The listing builds one solid part. Answer for the finished solid, in the listing's coordinates (mm). A direction names the side the tool comes from. Coordinates: 2 decimals unless noted, no trailing zeros. Order: outer loops, then holes, each group sorted by start corner. A loop starts at its lowest first (then second) coordinate and runs counter-clockwise, first axis right, second up. Notation, with made-up numbers: (-6, 23) -> (22, 23) arc R27 cw to (22, 50) -> close; hole circle Ø8 at (-23.75, 64.25). An arc over 180 degrees is marked (long way). Answer in a Markdown table with one row per item. Add a question column.
```python
from build123d import *

# Parameters (mm, degrees)
SKETCH1_W           = 88
SKETCH1_H           = 82
BOSS_EXTRUDE1_DEPTH = 3
SKETCH2_R           = 1.7
CUT_EXTRUDE1_DEPTH  = 4
SKETCH4_W           = 81.2
SKETCH4_H           = 75.2
SKETCH4_W_2         = 75.2
SKETCH4_H_2         = 69.2
BOSS_EXTRUDE2_DEPTH = 2
CUT_EXTRUDE5_START  = -3
SKETCH6_R           = 6
CUT_EXTRUDE5_DEPTH  = 3
SKETCH7_W           = 88
SKETCH7_H           = 3
BOSS_EXTRUDE3_DEPTH = 4
SKETCH8_R           = 3.75
BOSS_EXTRUDE4_DEPTH = 3


with BuildPart() as part:
    # Sketch1 → Boss-Extrude1 (new body)
    with BuildSketch(Plane(origin=(0, 0, 0), x_dir=(1, 0, 0), z_dir=(0, 1, 0))):
        Rectangle(SKETCH1_W, SKETCH1_H)
    extrude(amount=BOSS_EXTRUDE1_DEPTH)

    # Sketch2 → Cut-Extrude1 (cut, through all)
    with BuildSketch(Plane(origin=(0, 3, 0), x_dir=(1, 0, 0), z_dir=(0, 1, 0))):
        with Locations((-38, 35)):
            Circle(SKETCH2_R)
        with Locations((38, 35)):
            Circle(SKETCH2_R)
        with Locations((38, -35)):
            Circle(SKETCH2_R)
        with Locations((-38, -35)):
            Circle(SKETCH2_R)
    extrude(amount=-CUT_EXTRUDE1_DEPTH, mode=Mode.SUBTRACT)

    # Sketch4 → Boss-Extrude2 (add)
    with BuildSketch(Plane.XZ):
        Rectangle(SKETCH4_W, SKETCH4_H)
        Rectangle(SKETCH4_W_2, SKETCH4_H_2, mode=Mode.SUBTRACT)
    extrude(amount=BOSS_EXTRUDE2_DEPTH)

    # Sketch6 → Cut-Extrude5 (cut, through all)
    with BuildSketch(Plane(origin=(0, 3, 0), x_dir=(1, 0, 0), z_dir=(0, 1, 0)).offset(CUT_EXTRUDE5_START)):
        with Locations((-38, 35)):
            Circle(SKETCH6_R)
        with Locations((-38, -35)):
            Circle(SKETCH6_R)
        with Locations((38, -35)):
            Circle(SKETCH6_R)
        with Locations((38, 35)):
            Circle(SKETCH6_R)
    extrude(amount=-CUT_EXTRUDE5_DEPTH, mode=Mode.SUBTRACT)

    # Sketch7 → Boss-Extrude3 (add)
    with BuildSketch(Plane.XY.offset(41)):
        with Locations((0, 1.5)):
            Rectangle(SKETCH7_W, SKETCH7_H)
    extrude(amount=BOSS_EXTRUDE3_DEPTH)

    # Sketch8 → Boss-Extrude4 (add)
    with BuildSketch(Plane(origin=(0, 3, 0), x_dir=(1, 0, 0), z_dir=(0, 1, 0))):
        Polygon((-44, -41), (-44, -45), (44, -45), (44, -41), (44, 41), (-44, 41), align=None)
        with Locations((-38, 35)):
            Circle(SKETCH8_R, mode=Mode.SUBTRACT)
        with Locations((38, 35)):
            Circle(SKETCH8_R, mode=Mode.SUBTRACT)
        with Locations((-38, -35)):
            Circle(SKETCH8_R, mode=Mode.SUBTRACT)
        with Locations((38, -35)):
            Circle(SKETCH8_R, mode=Mode.SUBTRACT)
    extrude(amount=BOSS_EXTRUDE4_DEPTH)


solid = part.part
```
Q1. Determine the mould class of faces 6 (the face through (1, 3, -41)), 7 (the face through (-38.37, 1.52, -33.34)), 8 (the face through (0, -1, 34.6)), 9 (the face through (37.6, -1, 0)) for opening direction Z: +Z half, -Z half, draft (parallel to the pull), parting line (faces both ways), or undercut.
Q2. For faces 1 (the face through (-39.159, -0.986, -29.113)), 2 (the face through (-32.113, -0.986, 36.159)), 3 (the face through (-39.1, -1, 29.1)), 4 (the face through (32.113, -0.986, -36.159)), 5 (the face through (-41.746, 4.479, -35.165)), determine the directions among +Z, -Z, +X, -X, +Y, -Y from which every point of the face is accessible in a straight line to the end or side of a thin tool.
Q3. Straight lines are drawn through the part: line 1 (X direction, y = 4.9, z = 35); line 2 (X direction, y = 1, z = 35); line 3 (Z direction, x = 38, y = 1.3). For each, find the intervals that lie inside material, in ascending order.
Q4. Given pin 1 (10 mm diameter, centred on x = 38, z = 35, fed in from -Y); pin 2 (1 mm diameter, centred on x = 5.5, y = -1, fed in from -Z); pin 3 (1.6 mm diameter, centred on y = -1, z = 7, fed in from -X), each flat-ended and moving along its own axis, determine where each tip first touches the part or whether it passes through.
Q5. A cutting plane is placed at B-B (x = 2). Determine the outline of the cut face in (y, z).
Q6. A cutting plane is placed at A-A (z = -4). Determine the outline of the cut face in (x, y), then the cut area to 3 significant figures.
Returned:
| question | item | result |
|---|---|---|
| 1 | face 6 | -Z half |
| 1 | face 7 | undercut |
| 1 | face 8 | undercut |
| 1 | face 9 | draft |
| 2 | face 1 | -Z, -Y |
| 2 | face 2 | -X, -Y |
| 2 | face 3 | +Z, -Y |
| 2 | face 4 | +X, -Y |
| 2 | face 5 | +Y |
| 3 | line 1 | x = -44 to -41.75, -34.25 to 34.25, 41.75 to 44 |
| 3 | line 2 | x = -44 to -39.7, -36.3 to 36.3, 39.7 to 44 |
| 3 | line 3 | z = -41 to -36.7, -33.3 to 33.3, 36.7 to 45 |
| 4 | pin 1 | stops at y = 0 |
| 4 | pin 2 | stops at z = -37.6 |
| 4 | pin 3 | stops at x = -40.6 |
| 5 | outline | (-2, -37.6) -> (0, -37.6) -> (0, -41) -> (6, -41) -> (6, 45) -> (0, 45) -> (0, 37.6) -> (-2, 37.6) -> (-2, 34.6) -> (0, 34.6) -> (0, -34.6) -> (-2, -34.6) -> close |
| 6 | outline | (-44, 0) -> (-40.6, 0) -> (-40.6, -2) -> (-37.6, -2) -> (-37.6, 0) -> (37.6, 0) -> (37.6, -2) -> (40.6, -2) -> (40.6, 0) -> (44, 0) -> (44, 6) -> (-44, 6) -> close |
| 6 | area | 540 mm² |
